Could you check a few things on this model? Use its own coordinates, in mm. Face numbers are marked on the shaded views. A direction names the side the tool comes from. Coordinates: 2 decimals unless noted, no trailing zeros. Write each loop counter-clockwise with the first axis right and the second up, starting at its lowest first coordinate (ties: lowest second). Pieces come first, ordered by that corner, then holes.
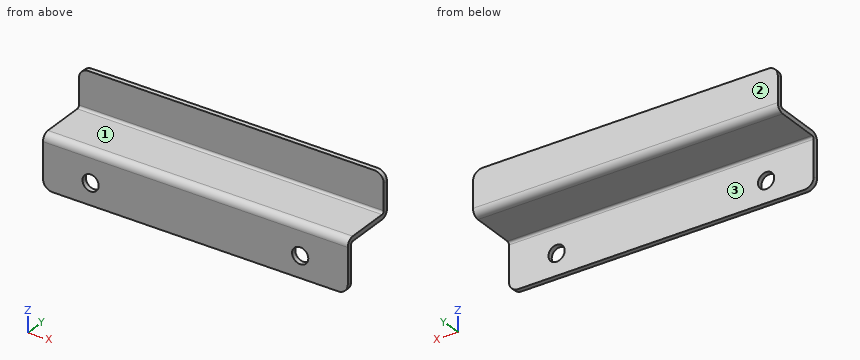
```python
from build123d import *

# Parameters (mm, degrees)
BASE_FLANGE1_DEPTH = 50.8
SKETCH4_R          = 2.7051
CUT_EXTRUDE1_DEPTH = 2.54
FILLET1_R          = 3.175


# Sheet-metal steps are written as plain solids
with BuildPart() as part:
    # Sketch1 → Base-Flange1 (new, symmetric)
    with BuildSketch(Plane(origin=(0, 0, 0), x_dir=(0, 0, -1), z_dir=(1, 0, 0))):
        with BuildLine():
            Line((-12.7, 17.4752), (-0.8128, 17.4752))
            ThreePointArc((-0.8128, 17.4752), (-0.238063608, 17.237136392), (0, 16.6624))
            Line((0, 16.6624), (0, 2.4003))
            ThreePointArc((0, 2.4003), (0.703031593, 0.703031593), (2.4003, 0))
            Line((2.4003, 0), (17.4752, 0))
            Line((17.4752, 0), (17.4752, 1.5875))
            Line((17.4752, 1.5875), (2.4003, 1.5875))
            ThreePointArc((2.4003, 1.5875), (1.825563608, 1.825563608), (1.5875, 2.4003))
            Line((1.5875, 2.4003), (1.5875, 16.6624))
            ThreePointArc((1.5875, 16.6624), (0.884468407, 18.359668407), (-0.8128, 19.0627))
            Line((-0.8128, 19.0627), (-12.7, 19.0627))
            Line((-12.7, 19.0627), (-12.7, 17.4752))
        make_face()
    extrude(amount=BASE_FLANGE1_DEPTH, both=True)

    # Sketch4 → Cut-Extrude1 (cut)
    with BuildSketch(Plane.XZ):
        with Locations(Location((34.93262, -10.3124, 0), (0, 0, 270))):
            Circle(SKETCH4_R)
        with Locations(Location((-34.925, -10.3124, 0), (0, 0, 270))):
            Circle(SKETCH4_R)
    extrude(amount=-CUT_EXTRUDE1_DEPTH, mode=Mode.SUBTRACT)

    # Fillet1
    fillet1_edges = [part.edges().sort_by_distance(p)[0] for p in [
        (-50.8, 0.79375, -17.4752),
        (-50.8, 18.26895, 12.7),
        (50.8, 0.79375, -17.4752),
        (50.8, 18.26895, 12.7),
    ]]
    fillet(fillet1_edges, radius=FILLET1_R)


solid = part.part
```
1. I want a section at B-B on z = -10.5. Please give me the cut outline in (x, y), plus the area to 3 significant figures.
Verdict:
outline: (-50.8, 0) - (-37.62, 0) - (-37.62, 1.59) - (-50.8, 1.59) - close; (-32.23, 0) - (32.23, 0) - (32.23, 1.59) - (-32.23, 1.59) - close; (37.63, 0) - (50.8, 0) - (50.8, 1.59) - (37.63, 1.59) - close
area: 144 mm2
2. I want a section at C-C on y = 12.25. Please give me the cut outline in (x, z).
Verdict:
outline: (-50.8, -1.59) - (50.8, -1.59) - (50.8, 0) - (-50.8, 0) - close
3. For pin 1 (8 mm diameter, centred on x = -27, z = 5, fed in from -Y); pin 2 (12 mm diameter, centred on x = 7.5, z = 5.5, fed in from -Y); pin 3 (7 mm diameter, centred on x = -17, y = 10.5, fed in from +Z), each with a flat end and sliding along its axis, tell me the tip position at first contact or that it passes through.
Verdict:
pin 1: stops at y = 17.48
pin 2: stops at y = 0.93
pin 3: stops at z = 0
4. I want a section at D-D on z = 2. Please give me the cut outline in (x, y).
Verdict:
outline: (-50.8, 17.48) - (50.8, 17.48) - (50.8, 19.06) - (-50.8, 19.06) - close
5. On a 3-axis mill with a long thin cutter (end or side, diameter ignored), from which of +Z, -Z, +X, -X, +Y, -Y can I reach the whole of each face in a straight line? I mean the marked faces 1, 2 and 3. Say none if no direction works.
Verdict:
face 1: +Z, +X, -X, -Y
face 2: +Z, -Z, +X, -X, +Y
face 3: -Z, +X, -X, +Y
6. Please list where these lines run through material, in increasing order: line 1 along Y through (x, z) = (6, 5.5); line 2 along Y through (x, z) = (19, -15.5); line 3 along Z through (x, y) = (-16.5, 10.5).
Verdict:
line 1: y = 17.48 to 19.06
line 2: y = 0 to 1.59
line 3: z = -1.59 to 0
7. I want a section at A-A on x = 21. Please give me the cut outline in (y, z), plus the area to 3 significant figures.
Verdict:
outline: (0, -17.48) - (1.59, -17.48) - (1.59, -2.4) arc R0.81 cw to (2.4, -1.59) - (16.66, -1.59) arc R2.4 ccw to (19.06, 0.81) - (19.06, 12.7) - (17.48, 12.7) - (17.48, 0.81) arc R0.81 cw to (16.66, 0) - (2.4, 0) arc R2.4 ccw to (0, -2.4) - close
area: 73.5 mm2
